Verification items for the finished model (mm, model axes). Face numbers are marked on the shaded views. A direction names the side the tool comes from. Give positions to 0.01 mm unless a question says otherwise; leave off trailing zeros. Order: outer loops, then holes, each group sorted by start corner. A loop starts at its lowest first (then second) coordinate and runs counter-clockwise, first axis right, second up. Notation, with made-up numbers: (38.5, -17) -> (89.5, -17) arc R32 ccw to (89.5, 9) -> close; hole circle Ø5 at (85.5, 53.5). An arc over 180 degrees is marked (long way). Write each question's results on one line, items separated by ' | '. Start each with the question number.
1. Set-up check for the marked faces 1, 2 and 3: record each of +Z, -Z, +X, -X, +Y, -Y from which the full face is reachable in a straight line by a thin tool's end or side.
2. Cross-section at A-A, the plane y = 0. Enter the section's corners in (x, z), then the cut area to 3 significant figures.
3. Material ranges on L1, parallel to X at y = -8.5, z = -3; L2, parallel to Y at x = 145, z = 0; L3, parallel to Z at x = 131, y = 1.5, recorded low to high. Write a range as from..to.
4. Depth check by flat-ended pin: pin 1 Ø8 at (x, z) = (68.5, -12.5) entering from -Y; pin 2 Ø4 at (x, y) = (-7, 1.5) entering from +Z; pin 3 Ø6 at (x, z) = (9, 3.5) entering from +Y. Enter the tip coordinate at first touch or a pass-through.
5. Cross-section at C-C, the plane x = 12.5. Enter the section's corners in (y, z).
6. Cross-section at D-D, the plane x = 33. Enter the section's corners in (y, z), then the cut area to 3 significant figures.
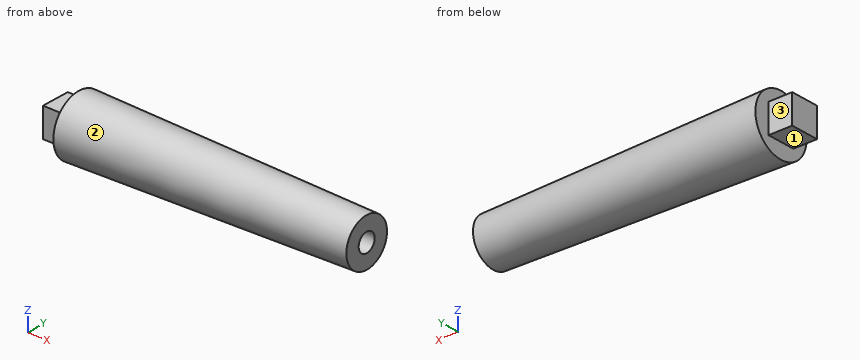
from build123d import *

# Parameters (mm, degrees)
SKETCH2_W           = 15.5
SKETCH2_H           = 15.5
BOSS_EXTRUDE1_DEPTH = 12.7
SKETCH3_R           = 5
CUT_EXTRUDE1_DEPTH  = 26


with BuildPart() as part:
    # Sketch1 → Revolve1 (revolve)
    with BuildSketch(Plane.XY, mode=Mode.PRIVATE) as revolve1_sk:
        Polygon((0, 0), (0, 16), (155, 12.7), (155, 0), align=None)
    revolve(revolve1_sk.sketch.rotate(Axis((155, 0, 0), (-1, 0, 0)), 90), axis=Axis((155, 0, 0), (-1, 0, 0)))

    # Sketch2 → Boss-Extrude1 (add)
    with BuildSketch(Plane.ZY):
        Rectangle(SKETCH2_W, SKETCH2_H)
    extrude(amount=BOSS_EXTRUDE1_DEPTH)

    # Sketch3 → Cut-Extrude1 (cut)
    with BuildSketch(Plane(origin=(155, 0, 0), x_dir=(0, 0, -1), z_dir=(1, 0, 0))):
        Circle(SKETCH3_R)
    extrude(amount=-CUT_EXTRUDE1_DEPTH, mode=Mode.SUBTRACT)


solid = part.part
Results below:
1) face 1: -Z, -X, +Y, -Y | face 2: +X | face 3: +Z, -Z, -X, +Y
2) outline: (-12.7, -7.75) -> (0, -7.75) -> (0, -16) -> (155, -12.7) -> (155, -5) -> (129, -5) -> (129, 5) -> (155, 5) -> (155, 12.7) -> (0, 16) -> (0, 7.75) -> (-12.7, 7.75) -> close | area: 4,390 mm²
3) L1: x = 0..155 | L2: y = -12.91..-5, 5..12.91 | L3: z = -13.13..-4.77, 4.77..13.13
4) pin 1: stops at y = -11.8 | pin 2: stops at z = 7.75 | pin 3: stops at y = 15.82
5) outline: circle Ø31.47 at (0, 0)
6) outline: circle Ø30.59 at (0, 0) | area: 735 mm²
